Verification items for the finished model (mm, model axes). Round coordinates to 2 decimals unless told otherwise and drop trailing zeros. Loops run counter-clockwise (first coordinate to the right, second up) from the corner with the lowest first, then second, coordinate; pieces in that order, holes last. Notation, with made-up numbers: M -37,64.5 L -3,64.5 A15 cw -3,72.5 Z; hole C -5.5,-27 d1. An arc over 180 degrees is marked long. Answer as CSV lines item,"result".
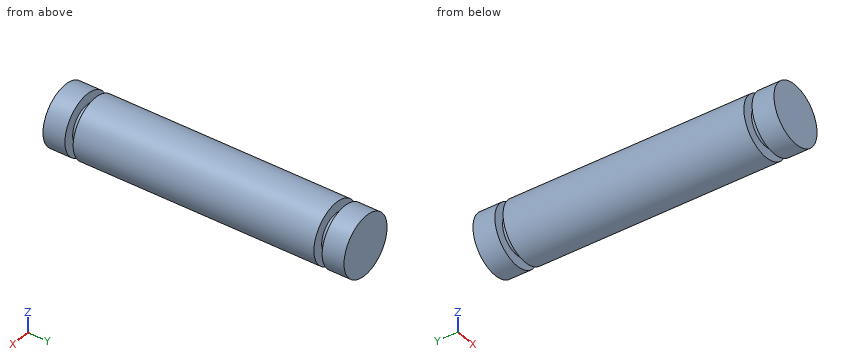
```python
from build123d import *

# Parameters (mm, degrees)
SKETCH2_R           = 2.5
BOSS_EXTRUDE1_DEPTH = 25
SKETCH3_W           = 0.9
SKETCH3_H           = 0.68


with BuildPart() as part:
    # Sketch2 → Boss-Extrude1 (new body)
    with BuildSketch(Plane(origin=(0, 0, 0), x_dir=(1, 0, 0), z_dir=(0, 1, 0))):
        Circle(SKETCH2_R)
    extrude(amount=BOSS_EXTRUDE1_DEPTH)

    # Sketch3 → Cut-Revolve1 (revolve, cut)
    with BuildSketch(Plane(origin=(0, 0, 0), x_dir=(0, 0, -1), z_dir=(1, 0, 0))):
        with Locations((-2.05, 2.16)):
            Rectangle(SKETCH3_W, SKETCH3_H)
        with Locations((-2.05, 22.84)):
            Rectangle(SKETCH3_W, SKETCH3_H)
    revolve(axis=Axis((0, 0, 0), (0, 1, 0)), mode=Mode.SUBTRACT)


solid = part.part
```
1) Section check D-D (y = 7.25). Record the cut outline in (x, z).
Here are the results:
outline,"C 0,0 d5"
2) Section check B-B (x = 0). Record the cut outline in (y, z), plus the area to 3 significant figures.
Here are the results:
outline,"M 0,-2.5 L 1.82,-2.5 L 1.82,-1.6 L 2.5,-1.6 L 2.5,-2.5 L 22.5,-2.5 L 22.5,-1.6 L 23.18,-1.6 L 23.18,-2.5 L 25,-2.5 L 25,2.5 L 23.18,2.5 L 23.18,1.6 L 22.5,1.6 L 22.5,2.5 L 2.5,2.5 L 2.5,1.6 L 1.82,1.6 L 1.82,2.5 L 0,2.5 Z"
area,"123 mm^2"
3) Material ranges on probe 1 along Y at (x, z) = (1.35, -1.7); probe 2 along Z at (x, y) = (0.15, 15), recorded low to high.
Here are the results:
probe 1,"y = 0 to 1.82, 2.5 to 22.5, 23.18 to 25"
probe 2,"z = -2.5 to 2.5"
4) Go/stop test with flat-tipped pins: pin 1 (1.5 mm diameter, centred on y = 21, z = 1.5, fed in from +X); pin 2 (1 mm diameter, centred on x = 2, y = 17, fed in from -Z). Record where each tip stops, or that it passes through.
Here are the results:
pin 1,"stops at x = 2.38"
pin 2,"stops at z = -2"
5) Section check C-C (z = 2.2). Record the cut outline in (x, y), plus the area to 3 significant figures.
Here are the results:
outline,"M -1.19,0 L 1.19,0 L 1.19,1.82 L -1.19,1.82 Z; M -1.19,2.5 L 1.19,2.5 L 1.19,22.5 L -1.19,22.5 Z; M -1.19,23.18 L 1.19,23.18 L 1.19,25 L -1.19,25 Z"
area,"56.1 mm^2"
6) Section check A-A (x = 2). Record the cut outline in (y, z).
Here are the results:
outline,"M 0,-1.5 L 1.82,-1.5 L 1.82,1.5 L 0,1.5 Z; M 2.5,-1.5 L 22.5,-1.5 L 22.5,1.5 L 2.5,1.5 Z; M 23.18,-1.5 L 25,-1.5 L 25,1.5 L 23.18,1.5 Z"
